The model under review builds one solid part; all positions refer to its coordinate system, in mm. A direction names the side the tool comes from. Give positions to 0.01 mm unless a question says otherwise; leave off trailing zeros. Order: outer loops, then holes, each group sorted by start corner. A loop starts at its lowest first (then second) coordinate and runs counter-clockwise, first axis right, second up.
```python
from build123d import *

# Parameters (mm, degrees)
SKETCH1_W           = 80
SKETCH1_H           = 80
BOSS_EXTRUDE1_DEPTH = 3
FILLET1_R           = 3
SKETCH2_R           = 2
CUT_EXTRUDE1_DEPTH  = 3
SKETCH3_R           = 35
CUT_EXTRUDE2_DEPTH  = 3
BOSS_EXTRUDE2_START = 10
SKETCH4_R           = 38.5
SKETCH4_R_2         = 35
BOSS_EXTRUDE2_DEPTH = 10
BOSS_EXTRUDE3_START = 3
SKETCH5_R           = 38.5
BOSS_EXTRUDE3_DEPTH = 3
SKETCH6_R           = 25
CUT_EXTRUDE3_DEPTH  = 3
SKETCH7_R           = 28.5
SKETCH7_R_2         = 25
BOSS_EXTRUDE4_DEPTH = 5
CHAMFER1_SIZE       = 2
CHAMFER2_SIZE       = 2


with BuildPart() as part:
    # Sketch1 → Boss-Extrude1 (new body)
    with BuildSketch(Plane(origin=(0, 0, 0), x_dir=(1, 0, 0), z_dir=(0, 1, 0))):
        Rectangle(SKETCH1_W, SKETCH1_H)
    extrude(amount=BOSS_EXTRUDE1_DEPTH)

    # Fillet1
    fillet1_edges = [part.edges().sort_by_distance(p)[0] for p in [
        (40, 1.5, 40),
        (-40, 1.5, 40),
        (-40, 1.5, -40),
        (40, 1.5, -40),
    ]]
    fillet(fillet1_edges, radius=FILLET1_R)

    # Sketch2 → Cut-Extrude1 (cut)
    with BuildSketch(Plane(origin=(0, 3, 0), x_dir=(1, 0, 0), z_dir=(0, 1, 0))):
        with Locations(Location((-36, 36, 0), (0, 0, 270))):
            Circle(SKETCH2_R)
        with Locations(Location((36, 36, 0), (0, 0, 270))):
            Circle(SKETCH2_R)
        with Locations(Location((-36, -36, 0), (0, 0, 270))):
            Circle(SKETCH2_R)
        with Locations(Location((36, -36, 0), (0, 0, 270))):
            Circle(SKETCH2_R)
    extrude(amount=-CUT_EXTRUDE1_DEPTH, mode=Mode.SUBTRACT)

    # Sketch3 → Cut-Extrude2 (cut)
    with BuildSketch(Plane(origin=(0, 3, 0), x_dir=(1, 0, 0), z_dir=(0, 1, 0))):
        with Locations(Location((0, 0, 0), (0, 0, 270))):
            Circle(SKETCH3_R)
    extrude(amount=-CUT_EXTRUDE2_DEPTH, mode=Mode.SUBTRACT)

    # Sketch4 → Boss-Extrude2 (add)
    with BuildSketch(Plane(origin=(0, 3, 0), x_dir=(1, 0, 0), z_dir=(0, 1, 0)).offset(BOSS_EXTRUDE2_START)):
        with Locations(Location((0, 0, 0), (0, 0, 270))):
            Circle(SKETCH4_R)
        with Locations(Location((0, 0, 0), (0, 0, 270))):
            Circle(SKETCH4_R_2, mode=Mode.SUBTRACT)
    extrude(amount=-BOSS_EXTRUDE2_DEPTH)

    # Sketch5 → Boss-Extrude3 (add)
    with BuildSketch(Plane(origin=(0, 13, 0), x_dir=(1, 0, 0), z_dir=(0, 1, 0)).offset(BOSS_EXTRUDE3_START)):
        with Locations(Location((0, 0, 0), (0, 0, 270))):
            Circle(SKETCH5_R)
    extrude(amount=-BOSS_EXTRUDE3_DEPTH)

    # Sketch6 → Cut-Extrude3 (cut)
    with BuildSketch(Plane(origin=(0, 16, 0), x_dir=(1, 0, 0), z_dir=(0, 1, 0))):
        with Locations(Location((0, 0, 0), (0, 0, 270))):
            Circle(SKETCH6_R)
    extrude(amount=-CUT_EXTRUDE3_DEPTH, mode=Mode.SUBTRACT)

    # Sketch7 → Boss-Extrude4 (add)
    with BuildSketch(Plane.XZ.offset(-13)):
        with Locations(Location((0, 0, 0), (0, 0, 90))):
            Circle(SKETCH7_R)
        with Locations(Location((0, 0, 0), (0, 0, 90))):
            Circle(SKETCH7_R_2, mode=Mode.SUBTRACT)
    extrude(amount=BOSS_EXTRUDE4_DEPTH)

    # Chamfer1
    chamfer1_edges = [part.edges().sort_by_distance(p)[0] for p in [
        (0, 13, -28.5),
    ]]
    chamfer(chamfer1_edges, length=CHAMFER1_SIZE)

    # Chamfer2
    # the kernel refuses this chamfer: 2 mm, written as the material it adds along each edge
    with BuildSketch(Plane(origin=(0, 3, 0), x_dir=(0, 0, 1), z_dir=(-1, 0, 0))) as chamfer2_piece_1_section:
        Polygon((38.5 + CHAMFER2_SIZE, 0), (38.5, CHAMFER2_SIZE), (38.5, 0), align=None)
    chamfer2_piece_1 = revolve(axis=Axis((0, 3, 0), (0, 1, 0)), mode=Mode.PRIVATE)
    chamfer2_piece_1 = split(chamfer2_piece_1, bisect_by=Plane(origin=(0, 3.942538478, -40), z_dir=(0, 0, 1)), keep=Keep.TOP, mode=Mode.PRIVATE)
    chamfer2_piece_1 = split(chamfer2_piece_1, bisect_by=Plane(origin=(-40, 3.942538478, -39.442538478), z_dir=(1, 0, 0)), keep=Keep.TOP, mode=Mode.PRIVATE)
    chamfer2_piece_1 = split(chamfer2_piece_1, bisect_by=Plane(origin=(40, 3.942538478, -39.442538478), z_dir=(-1, 0, 0)), keep=Keep.TOP, mode=Mode.PRIVATE)
    chamfer2_piece_1 = split(chamfer2_piece_1, bisect_by=Plane(origin=(0, 3.942538478, 40), z_dir=(0, 0, -1)), keep=Keep.TOP, mode=Mode.PRIVATE)
    add(chamfer2_piece_1)


solid = part.part
```
1. To check wall thickness, follow line 1 (X direction, y = 2.45, z = -36); line 2 (X direction, y = 9, z = 0); line 3 (Z direction, x = -10.5, y = 12.5). State the ranges of each line that lie inside material, in increasing order.
2. Draft analysis for pull direction X (two halves, no side actions). For faces 6 (the cylindrical face through (39.1, 1.52, 39.14)), 7 (the cylindrical face through (27.82, 9.52, -6.18)), 8 (the flat face through (25.2, 8, -0.1)), 9 (the flat face through (-1, 2, -40)), state which applies: pulls with the +X half, pulls with the -X half, needs draft (parallel to the pull), parting line crosses it, or undercut.
3. Take a section at C-C (z = -36). Count the separate pieces of the cut face and the enclosed holes in it, and give its area (3 significant figures).
4. For faces 1 (the flat face through (31, 3, 31)), 2 (the flat face through (29, 13, -11)), 3 (the flat face through (-32, 3, 31)), 4 (the cylindrical face through (-37.584, 10.577, -8.346)), 5 (the flat face through (-31, 3, -31)), list the 3-axis set-ups (+Z, -Z, +X, -X, +Y, -Y) from which the entire face can be reached by the end or side of a thin tool; tool diameter is ignored.
5. Take a section at B-B (x = 0). Write out the cut boundary in (y, z).
6. Insertion check: pin 1 (1.5 mm diameter, centred on y = 12, z = -9, fed in from -X); pin 2 (8 mm diameter, centred on x = -23.5, y = 13.5, fed in from -Z); pin 3 (21 mm diameter, centred on x = 2.5, z = 3.5, fed in from -Y); pin 4 (5 mm diameter, centred on x = 36, z = -36, fed in from +Y). Each pin has a flat end and moves straight along its axis. Give the tip position at first contact, or say it passes through.
7. Take a section at A-A (z = 0). Write out the cut boundary in (x, y), and give its area (3 significant figures).
Answer:
1. line 1: x = -40 to -38, -34 to 34, 38 to 40
1. line 2: x = -38.5 to -35, -28.5 to -25, 25 to 28.5, 35 to 38.5
1. line 3: z = -37.04 to -33.39, -28.1 to -22.69, 22.69 to 28.1, 33.39 to 37.04
2. face 6: pulls with the +X half
2. face 7: undercut
2. face 8: undercut
2. face 9: needs draft
3. separate pieces: 3
3. enclosed holes: 0
3. area: 581 mm2
4. face 1: +Z, +X, +Y
4. face 2: -Y
4. face 3: +Z, -X, +Y
4. face 4: +Y
4. face 5: -Z, -X, +Y
5. outline: (0, -40) - (3.5, -40) - (5, -38.5) - (16, -38.5) - (16, -25) - (8, -25) - (8, -28.5) - (11, -28.5) - (13, -30.5) - (13, -35) - (0, -35) - close; (0, 35) - (13, 35) - (13, 30.5) - (11, 28.5) - (8, 28.5) - (8, 25) - (16, 25) - (16, 38.5) - (5, 38.5) - (3.5, 40) - (0, 40) - close
6. pin 1: stops at x = -37.61
6. pin 2: stops at z = -33.2
6. pin 3: passes through
6. pin 4: stops at y = 3
7. outline: (-40, 0) - (-35, 0) - (-35, 13) - (-30.5, 13) - (-28.5, 11) - (-28.5, 8) - (-25, 8) - (-25, 16) - (-38.5, 16) - (-38.5, 5) - (-40, 3.5) - close; (25, 8) - (28.5, 8) - (28.5, 11) - (30.5, 13) - (35, 13) - (35, 0) - (40, 0) - (40, 3.5) - (38.5, 5) - (38.5, 16) - (25, 16) - close
7. area: 224 mm2
